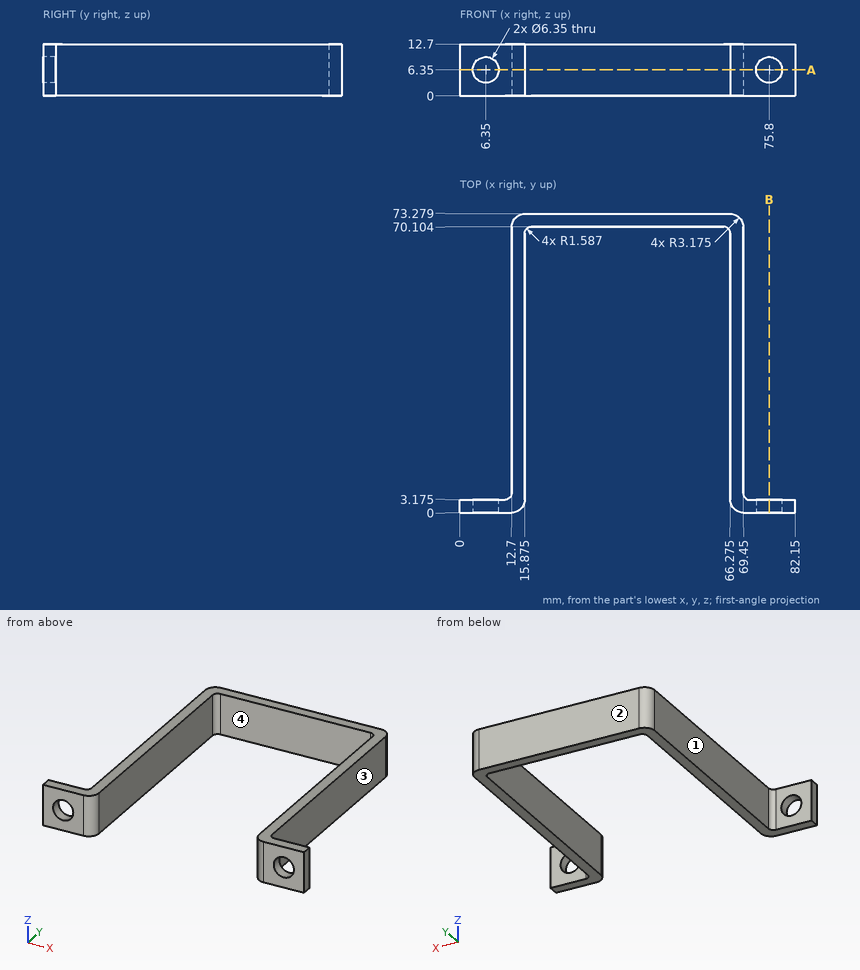
The drawing under review shows one solid part. Ordinate dimensions are in mm from its lowest x, y, z. Give positions to 0.01 mm unless a question says otherwise; leave off trailing zeros. Loops run counter-clockwise (first coordinate to the right, second up) from the corner with the lowest first, then second, coordinate; pieces in that order, holes last. Notation, with made-up numbers: M -32.5,11 L 5.5,11 A31 cw 5.5,42 Z; hole C 51.25,51 d5. An arc over 180 degrees is marked long. One line per item, written item: value. Start each with the question number.
Q1. Clearance check with flat-ended pins moving along their axes: pin 1 Ø5.5 at (x, z) = (74.5, 8.5) entering from +Y (1 decimal); pin 2 Ø6.5 at (y, z) = (43.5, 8) entering from -X; pin 3 Ø10 at (x, y) = (8.5, 61.5) entering from +Z; pin 4 Ø6 at (y, z) = (33, 7.5) entering from +X. State where each tip first meets the part, or that it passes through.
Q2. Add section A-A (z = 6.35). Count the separate pieces of the cut face and the enclosed holes in it.
Q3. For L1, parallel to Z at x = 6.35, y = 1.85 (1 decimal); L2, parallel to Y at x = 42, z = 9 (1 decimal); L3, parallel to Z at x = 75, y = 1, list the stretches that pass through material, from the lowest coordinate up.
Q4. Add section B-B (x = 75.8). Give the boundary of the cut face in (y, z) (1 decimal).
Q5. Draft analysis for pull direction X (two halves, no side actions). For the marked faces 1, 2, 3 and 4, state which applies: released by +X, released by -X, zero draft, split by the parting line, or undercut.
Reply:
1. pin 1: y = 3.2
1. pin 2: x = 12.7
1. pin 3: z = 12.7
1. pin 4: x = 69.45
2. separate pieces: 3
2. enclosed holes: 0
3. L1: 0 to 3.2, 9.5 to 12.7
3. L2: 70.1 to 73.3
3. L3: 0 to 3.28, 9.42 to 12.7
4. outline: M 0,0 L 3.2,0 L 3.2,3.2 L 0,3.2 Z; M 0,9.5 L 3.2,9.5 L 3.2,12.7 L 0,12.7 Z
5. face 1: released by -X
5. face 2: zero draft
5. face 3: released by +X
5. face 4: undercut
